from build123d import *

# Parameters (mm, degrees)
SKETCH4_R          = 3.25
CUT_EXTRUDE1_DEPTH = 10
FILLET2_R          = 0.5


with BuildPart() as part:
    # Sketch3 → Revolve1 (revolve)
    with BuildSketch(Plane.XY, mode=Mode.PRIVATE) as revolve1_sk:
        Polygon((0, 34.25), (0, 60), (2.5, 60), (2.5, 36.75), (18, 36.75), (18, 34.25), align=None)
    revolve(revolve1_sk.sketch.rotate(Axis((0, 0, 0), (1, 0, 0)), 90), axis=Axis((0, 0, 0), (1, 0, 0)))

    # Sketch4 → Cut-Extrude1 (cut)
    with BuildSketch(Plane.ZY):
        with Locations((30.329719018, 41.74527691)):
            Circle(SKETCH4_R)
        with Locations((0, 51.6)):
            Circle(SKETCH4_R)
        with Locations((49.074516241, 15.94527691)):
            Circle(SKETCH4_R)
        with Locations((49.074516241, -15.94527691)):
            Circle(SKETCH4_R)
        with Locations((30.329719018, -41.74527691)):
            Circle(SKETCH4_R)
        with Locations((0, -51.6)):
            Circle(SKETCH4_R)
        with Locations((-30.329719018, -41.74527691)):
            Circle(SKETCH4_R)
        with Locations((-49.074516241, -15.94527691)):
            Circle(SKETCH4_R)
        with Locations((-49.074516241, 15.94527691)):
            Circle(SKETCH4_R)
        with Locations((-30.329719018, 41.74527691)):
            Circle(SKETCH4_R)
    extrude(amount=-CUT_EXTRUDE1_DEPTH, mode=Mode.SUBTRACT)

    # Fillet2
    fillet2_edges = [part.edges().sort_by_distance(p)[0] for p in [
        (2.5, 0, -36.75),
    ]]
    fillet(fillet2_edges, radius=FILLET2_R)


solid = part.part
Could you check a few things on this model? Use its own coordinates, in mm. A direction names the side the tool comes from. Give positions to 0.01 mm unless a question says otherwise; leave off trailing zeros. Order: outer loops, then holes, each group sorted by start corner. A loop starts at its lowest first (then second) coordinate and runs counter-clockwise, first axis right, second up.
1. Thinking about a two-plate mould opening in Z: for faces 1 (the cylindrical face through (1.232, 13.968, 46.495)), 2 (the flat face through (18, -17, -30)), 3 (the cylindrical face through (1.27, -50.59, 32.26)), which applies, +Z half, -Z half, draft (parallel to the pull), parting line (faces both ways), or undercut?
Answers below:
face 1: undercut
face 2: draft
face 3: parting line
2. Suppose I cut it at D-D (x = 10.5). Write out the boundary of the cut face in (y, z).
Answers below:
outline: circle Ø73.5 at (0, 0); hole circle Ø68.5 at (0, 0)
3. Which directions (+Z, -Z, +X, -X, +Y, -Y) give clear straight access to the entire face, cutting with the end or side of a thin tool? Please do faces 4 (the cylindrical face through (1.23, 39.77, -32.91)), 5 (the cylindrical face through (10.605, 35.876, -7.967)).
Answers below:
face 4: +X, -X
face 5: +X
4. For pin 1 (1 mm diameter, centred on x = 2.5, z = 29.5, fed in from -Y); pin 2 (4 mm diameter, centred on y = 15.95, z = 49.07, fed in from -X); pin 3 (1.5 mm diameter, centred on x = 5.5, y = -11.5, fed in from -Z); pin 4 (4 mm diameter, centred on x = 11, y = -20.5, fed in from +Z), each with a flat end and sliding along its axis, tell me the tip position at first contact or that it passes through.
Answers below:
pin 1: stops at y = -52.53
pin 2: passes through
pin 3: stops at z = -35.14
pin 4: stops at z = 31.75
5. Suppose I cut it at B-B (z = 0). Write out the boundary of the cut face in (x, y).
Answers below:
outline: (0, -60) - (2.5, -60) - (2.5, -54.85) - (0, -54.85) - close; (0, -48.35) - (2.5, -48.35) - (2.5, -37.25) arc R0.5 cw to (3, -36.75) - (18, -36.75) - (18, -34.25) - (0, -34.25) - close; (0, 34.25) - (18, 34.25) - (18, 36.75) - (3, 36.75) arc R0.5 cw to (2.5, 37.25) - (2.5, 48.35) - (0, 48.35) - close; (0, 54.85) - (2.5, 54.85) - (2.5, 60) - (0, 60) - close
6. I need wall thicknesses on L1, parallel to Y at x = 4.5, z = -0.5; L2, parallel to Z at x = 11, y = 1; L3, parallel to X at y = -53, z = 7. Which ranges of each line are inside material? Lowest first, please.
Answers below:
L1: y = -36.75 to -34.25, 34.25 to 36.75
L2: z = -36.74 to -34.24, 34.24 to 36.74
L3: x = 0 to 2.5
7. Suppose I cut it at C-C (z = 50). Write out the boundary of the cut face in (x, y), plus the area to 3 significant figures.
Answers below:
outline: (0, -33.17) - (2.5, -33.17) - (2.5, -19.06) - (0, -19.06) - close; (0, -12.83) - (2.5, -12.83) - (2.5, 12.83) - (0, 12.83) - close; (0, 19.06) - (2.5, 19.06) - (2.5, 33.17) - (0, 33.17) - close
area: 135 mm2
8. Suppose I cut it at A-A (y = 0). Write out the boundary of the cut face in (x, z), plus the area to 3 significant figures.
Answers below:
outline: (0, -60) - (2.5, -60) - (2.5, -37.25) arc R0.5 cw to (3, -36.75) - (18, -36.75) - (18, -34.25) - (0, -34.25) - close; (0, 34.25) - (18, 34.25) - (18, 36.75) - (3, 36.75) arc R0.5 cw to (2.5, 37.25) - (2.5, 60) - (0, 60) - close
area: 206 mm2
